Read the model definition and answer for the solid it produces. Units are mm, in the model's axes. A direction names the side the tool comes from. Coordinates: 2 decimals unless noted, no trailing zeros. Write each loop counter-clockwise with the first axis right and the second up, starting at its lowest first coordinate (ties: lowest second). Pieces come first, ordered by that corner, then holes. Notation, with made-up numbers: (-39.5, 57) -> (-8.5, 57) arc R36 ccw to (-8.5, 93) -> close; hole circle Ø8 at (-40, 64.25). An arc over 180 degrees is marked (long way). Use CSV: the item, a comma, the result in double quotes.
from build123d import *

# Parameters (mm, degrees)
SZKIC1_W                          = 596
SZKIC1_H                          = 396
SZKIC1_R                          = 24
SZKIC1_R_2                        = 21
DODANIE_WYCI_GNI_CIE1_DEPTH       = 46
OTW_R_GWINTOWANY_M161_D           = 14
SZKIC5_R                          = 5
WYTNIJ_WYCI_GNI_CIE1_DEPTH        = 718.041142474
OTW_R_GWINTOWANY_M241_AT_2_COUNT  = 2
OTW_R_GWINTOWANY_M241_AT_2_PITCH  = 80
OTW_R_GWINTOWANY_M241_AT_3_COUNT  = 2
OTW_R_GWINTOWANY_M241_AT_3_PITCH  = 170
OTW_R_GWINTOWANY_M241_AT_4_COUNT  = 2
OTW_R_GWINTOWANY_M241_AT_4_PITCH  = 250
OTW_R_GWINTOWANY_M201_D           = 17.5
OTW_R_GWINTOWANY_M201_DEPTH       = 52.5
OTW_R_GWINTOWANY_M201_CSINK_D     = 20.05
OTW_R_GWINTOWANY_M201_CSINK_ANGLE = 90
OTW_R_GWINTOWANY_M201_TIP         = 5.257530416


with BuildPart() as part:
    # Szkic1 → Dodanie-wyciągnięcie1 (new body)
    # profile 1 of 5: a face of its own
    with BuildSketch(Plane(origin=(0, 0, 0), x_dir=(1, 0, 0), z_dir=(0, 1, 0))):
        with Locations((298, 198)):
            Rectangle(SZKIC1_W, SZKIC1_H)
        with Locations((560, 360)):
            Circle(SZKIC1_R, mode=Mode.SUBTRACT)
        with Locations((36, 360)):
            Circle(SZKIC1_R, mode=Mode.SUBTRACT)
        with Locations((560, 36)):
            Circle(SZKIC1_R, mode=Mode.SUBTRACT)
        with Locations((36, 36)):
            Circle(SZKIC1_R, mode=Mode.SUBTRACT)
    # profile 2 of 5: a face of its own
    with BuildSketch(Plane(origin=(0, 0, 0), x_dir=(1, 0, 0), z_dir=(0, 1, 0))):
        with Locations((36, 36)):
            Circle(SZKIC1_R)
        with Locations(Location((36, 36, 0), (0, 0, 270))):
            Circle(SZKIC1_R_2, mode=Mode.SUBTRACT)
    # profile 3 of 5: a face of its own
    with BuildSketch(Plane(origin=(0, 0, 0), x_dir=(1, 0, 0), z_dir=(0, 1, 0))):
        with Locations((560, 36)):
            Circle(SZKIC1_R)
        with Locations(Location((560, 36, 0), (0, 0, 270))):
            Circle(SZKIC1_R_2, mode=Mode.SUBTRACT)
    # profile 4 of 5: a face of its own
    with BuildSketch(Plane(origin=(0, 0, 0), x_dir=(1, 0, 0), z_dir=(0, 1, 0))):
        with Locations((560, 360)):
            Circle(SZKIC1_R)
        with Locations(Location((560, 360, 0), (0, 0, 270))):
            Circle(SZKIC1_R_2, mode=Mode.SUBTRACT)
    # profile 5 of 5: a face of its own
    with BuildSketch(Plane(origin=(0, 0, 0), x_dir=(1, 0, 0), z_dir=(0, 1, 0))):
        with Locations((36, 360)):
            Circle(SZKIC1_R)
        with Locations(Location((36, 360, 0), (0, 0, 270))):
            Circle(SZKIC1_R_2, mode=Mode.SUBTRACT)
    extrude(amount=-DODANIE_WYCI_GNI_CIE1_DEPTH)

    # Otwór gwintowany M161 (through all)
    with Locations(Plane(origin=(83, 0, -360), x_dir=(0, 0, 1), z_dir=(0, 1, 0))):
        with Locations((0, 0), (0, 430), (324, 0), (324, 430)):
            Hole(OTW_R_GWINTOWANY_M161_D / 2)

    # Szkic5 → Wytnij-wyciągnięcie1 (cut, through all)
    with BuildSketch(Plane.XY):
        with Locations((133, -23)):
            Circle(SZKIC5_R)
        with Locations((213, -23)):
            Circle(SZKIC5_R)
        with Locations(Location((463, -23, 0), (0, 0, 180))):
            Circle(SZKIC5_R)
        with Locations(Location((383, -23, 0), (0, 0, 180))):
            Circle(SZKIC5_R)
    extrude(amount=-WYTNIJ_WYCI_GNI_CIE1_DEPTH, mode=Mode.SUBTRACT)

    # Szkic6 → Otwór gwintowany M241 (revolve, cut)
    with BuildSketch(Plane(origin=(213, -23, 0), x_dir=(0, -1, 0), z_dir=(1, 0, 0))):
        Polygon((0, 0), (0, 41.3090365), (10.5, 35), (10.5, 1.525), (12.025, 0), align=None)
    otw_r_gwintowany_m241 = revolve(axis=Axis((213, -23, 6.35), (0, 0, -1)), mode=Mode.SUBTRACT)

    # Otwór gwintowany M241 at 2: Otwór gwintowany M241 ×2
    with Locations(*[(-i * OTW_R_GWINTOWANY_M241_AT_2_PITCH, 0, 0) for i in range(1, OTW_R_GWINTOWANY_M241_AT_2_COUNT)]):
        add(otw_r_gwintowany_m241, mode=Mode.SUBTRACT)

    # Otwór gwintowany M241 at 3: Otwór gwintowany M241 ×2
    with Locations(*[(i * OTW_R_GWINTOWANY_M241_AT_3_PITCH, 0, 0) for i in range(1, OTW_R_GWINTOWANY_M241_AT_3_COUNT)]):
        add(otw_r_gwintowany_m241, mode=Mode.SUBTRACT)

    # Otwór gwintowany M241 at 4: Otwór gwintowany M241 ×2
    with Locations(*[(i * OTW_R_GWINTOWANY_M241_AT_4_PITCH, 0, 0) for i in range(1, OTW_R_GWINTOWANY_M241_AT_4_COUNT)]):
        add(otw_r_gwintowany_m241, mode=Mode.SUBTRACT)

    # Lustro1: Otwór gwintowany M241 across plane
    add(otw_r_gwintowany_m241.mirror(Plane.XY.offset(-198)), mode=Mode.SUBTRACT)

    # Lustro1 copy 1 sketch → Lustro1 copy 1 (revolve, cut)
    with BuildSketch(Plane(origin=(133, -23, -396), x_dir=(0, -1, 0), z_dir=(1, 0, 0))):
        Polygon((0, 0), (0, -41.3090365), (10.5, -35), (10.5, -1.525), (12.025, 0), align=None)
    revolve(axis=Axis((133, -23, -402.35), (0, 0, -1)), mode=Mode.SUBTRACT)

    # Lustro1 copy 2 sketch → Lustro1 copy 2 (revolve, cut)
    with BuildSketch(Plane(origin=(383, -23, -396), x_dir=(0, -1, 0), z_dir=(1, 0, 0))):
        Polygon((0, 0), (0, -41.3090365), (10.5, -35), (10.5, -1.525), (12.025, 0), align=None)
    revolve(axis=Axis((383, -23, -402.35), (0, 0, -1)), mode=Mode.SUBTRACT)

    # Lustro1 copy 3 sketch → Lustro1 copy 3 (revolve, cut)
    with BuildSketch(Plane(origin=(463, -23, -396), x_dir=(0, -1, 0), z_dir=(1, 0, 0))):
        Polygon((0, 0), (0, -41.3090365), (10.5, -35), (10.5, -1.525), (12.025, 0), align=None)
    revolve(axis=Axis((463, -23, -402.35), (0, 0, -1)), mode=Mode.SUBTRACT)

    # Otwór gwintowany M201
    with Locations(Plane(origin=(298, -23, 0), x_dir=(1, 0, 0), z_dir=(0, 0, 1))):
        with Locations((0, 0)):
            CounterSinkHole(OTW_R_GWINTOWANY_M201_D / 2, OTW_R_GWINTOWANY_M201_CSINK_D / 2, depth=OTW_R_GWINTOWANY_M201_DEPTH, counter_sink_angle=OTW_R_GWINTOWANY_M201_CSINK_ANGLE)
            with Locations((0, 0, -(OTW_R_GWINTOWANY_M201_DEPTH + OTW_R_GWINTOWANY_M201_TIP / 2))):  # 118° drill point
                Cone(0, OTW_R_GWINTOWANY_M201_D / 2, OTW_R_GWINTOWANY_M201_TIP, mode=Mode.SUBTRACT)


solid = part.part
1. Each of these flat-tipped pins is pushed along its axis until it touches: pin 1 Ø25 at (x, z) = (36, -360) entering from +Y; pin 2 Ø19 at (x, y) = (383, -23) entering from +Z; pin 3 Ø24 at (x, y) = (463, -23) entering from +Z (3 decimals). Where does it stop, or does it pass through?
Solutions:
pin 1,"passes through"
pin 2,"stops at z = -35.6"
pin 3,"stops at z = -0.025"
2. Find the intervals of material crossed by line 1 along X through (y, z) = (-23, -223); line 2 along X through (y, z) = (-10, -36); line 3 along Z through (x, y) = (513, -14), in increasing order.
Solutions:
line 1,"x = 0 to 128, 138 to 208, 218 to 378, 388 to 458, 468 to 596"
line 2,"x = 0 to 15, 57 to 76, 90 to 506, 520 to 539, 581 to 596"
line 3,"z = -396 to -367, -353 to -43, -29 to 0"
3. A tool of negligible diameter and unlimited length cuts with its end or side. For faces 1 (the cylindrical face through (202.59, -21.63, -377.97)), 2 (the flat face through (596, -23, -195)), 3 (the cylindrical face through (143.25, -20.72, -18.03)), from which of +Z, -Z, +X, -X, +Y, -Y can it reach the whole face along a straight path? Write none if from no direction.
Solutions:
face 1,"-Z"
face 2,"+Z, -Z, +X, +Y, -Y"
face 3,"+Z"
4. For a pull along X with two mould halves and no side action, classify faces 4 (the flat face through (0, -23, -195)), 5 (the cylindrical face through (473.25, -20.72, -18.03)), 6 (the flat face through (294, -46, -201)), 7 (the cylindrical face through (539.5, -22.68, -364.55)) as pulls with the +X half, pulls with the -X half, needs draft (parallel to the pull), parting line crosses it, or undercut.
Solutions:
face 4,"pulls with the -X half"
face 5,"undercut"
face 6,"needs draft"
face 7,"undercut"
5. A cutting plane is placed at A-A (x = 49). Give the vertices of the cut face in (y, z), and give its area (3 significant figures).
Solutions:
outline,"(-46, -396) -> (0, -396) -> (0, -376.49) -> (-46, -376.49) -> close; (-46, -343.51) -> (0, -343.51) -> (0, -52.49) -> (-46, -52.49) -> close; (-46, -19.51) -> (0, -19.51) -> (0, 0) -> (-46, 0) -> close"
area,"15,200 mm^2"
